Work out the finished part from the listing and answer in its coordinate system (mm). A direction names the side the tool comes from. Round coordinates to 2 decimals unless told otherwise and drop trailing zeros. Order: outer loops, then holes, each group sorted by start corner. A loop starts at its lowest first (then second) coordinate and runs counter-clockwise, first axis right, second up. Notation, with made-up numbers: M 69.25,-12 L 110.25,-12 A36 ccw 110.25,23 Z; hole C 57,-22.75 d11. An arc over 180 degrees is marked long. Return JSON: item names as keys, results as strings.
from build123d import *

# Parameters (mm, degrees)
CYLINDER011_R             = 1
CYLINDER011_DEPTH         = 1
CYLINDER003_R             = 2.25
CYLINDER003_DEPTH         = 10
ARRAY_X_COUNT             = 2
ARRAY_X_PITCH             = 49.5
ARRAY_Z_COUNT             = 2
ARRAY_Z_PITCH             = 10
EXTRUDE003_DEPTH          = 20.2
CUT004_ROLL_ANGLE         = -90
CUT004_PLACEMENT_ANGLE    = 90
FUSION002_PLACEMENT_ANGLE = 7


with BuildPart() as cylinder011:
    # Cylinder011 → Cylinder011 (new body)
    with BuildSketch(Plane(origin=(80, 0, -1), x_dir=(1, 0, 0), z_dir=(0, 0, 1))):
        Circle(CYLINDER011_R)
    extrude(amount=CYLINDER011_DEPTH)


with BuildPart() as array:
    # Cylinder003 → Cylinder003 (new body)
    with BuildSketch(Plane.XZ):
        Circle(CYLINDER003_R)
    extrude(amount=CYLINDER003_DEPTH)

    # Array X: Array ×2


with BuildPart() as array_1:
    add(array.part)
    with Locations(*[(i * ARRAY_X_PITCH, 0, 0) for i in range(1, ARRAY_X_COUNT)]):
        add(array.part)

    # Array Z: Array ×2


with BuildPart() as array_2:
    add(array_1.part)
    with Locations(*[(0, 0, i * ARRAY_Z_PITCH) for i in range(1, ARRAY_Z_COUNT)]):
        add(array_1.part)


with BuildPart() as array_3:
    # Array placement: moved
    add(array_2.part.moved(Location((-56.5, 22, 5))))


with BuildPart() as servo_pan:
    # Sketch002 → Extrude003 (new body)
    with BuildSketch(Plane.XY):
        Polygon((-59.135985, 19.221684), (-52.235985, 19.221684), (-52.235985, 27.421684), (-11.035985, 27.421684), (-11.035985, 19.221684), (-4.135985, 19.221684), (-4.135985, 16.721684), (-11.035985, 16.721684), (-11.035985, -10.278316), (-52.235985, -10.278316), (-52.235985, 16.721684), (-59.135985, 16.721684), align=None)
    extrude(amount=EXTRUDE003_DEPTH)

    # Cut004: cut Array
    add(array_3.part, mode=Mode.SUBTRACT)


with BuildPart() as servo_pan_1:
    # Cut004 roll: moved
    add(servo_pan.part.rotate(Axis((0, 0, 0), (1, 0, 0)), CUT004_ROLL_ANGLE))


with BuildPart() as servo_pan_2:
    # Cut004 placement: moved
    add(servo_pan_1.part.moved(Location((90, 21, 27))).rotate(Axis((90, 21, 27), (0, 0, 1)), CUT004_PLACEMENT_ANGLE))

    # Fusion002: union Cylinder011
    add(cylinder011.part)


with BuildPart() as servo_pan_3:
    # Fusion002 placement: moved
    add(servo_pan_2.part.moved(Location((0.6, 9.75, 0))).rotate(Axis((0.6, 9.75, 0), (0, 0, -1)), FUSION002_PLACEMENT_ANGLE))


solid = servo_pan_3.part
Item 1: Which of the six approach directions +Z, -Z, +X, -X, +Y, -Y give full straight-line access (tool end or side, diameter ignored) to faces 1 (the cylindrical face through (80.874, -0.492, -0.715)), 2 (the flat face through (82, 13, 10.278)), 3 (the flat face through (76, -34, 10.278)), 4 (the flat face through (82, 13, 7.778))?
Output:
{"face 1": "-Z", "face 2": "+Z, +X, +Y", "face 3": "+Z, -X, -Y", "face 4": "-Z, +X, +Y"}
Item 2: Find section A-A (x = 88.25). Determine the outline of the cut face in (y, z).
Output:
{"outline": "M -14.89,-0.42 L 9.03,-0.42 L 9.03,7.78 L 11.68,7.78 L 11.68,10.28 L 9.03,10.28 L 9.03,37.28 L -14.89,37.28 Z; M 14.89,7.78 L 15.98,7.78 L 15.98,10.28 L 14.89,10.28 Z"}
Item 3: Consider line 1 along Z through (x, y) = (74, -21); line 2 along Z through (x, y) = (80.5, 11); line 3 along Y through (x, z) = (75, 18.5). Determine where each line is inside the solid, lowest interval first. Write a range as [from, to].
Output:
{"line 1": "z = [-0.42, 37.28]", "line 2": "z = [7.78, 10.28]", "line 3": "y = [-30.86, 10.65]"}
Item 4: The mould has two halves that part along X. Classify faces 5 (the flat face through (68.63, -8.93, 18.16)), 6 (the flat face through (79, -11, -0.422)), 7 (the cylindrical face through (75.011, 15.937, 9.011)), 8 (the flat face through (81.259, 9.885, 23.589)): pulls with the +X half, pulls with the -X half, needs draft (parallel to the pull), parting line crosses it, or undercut.
Output:
{"face 5": "pulls with the -X half", "face 6": "needs draft", "face 7": "undercut", "face 8": "pulls with the +X half"}
Item 5: Find section D-D (x = 79.75). Determine the outline of the cut face in (y, z).
Output:
{"outline": "M -38.39,7.78 L -37.91,7.78 L -37.91,10.28 L -38.39,10.28 Z; M -33.78,7.78 L -31.44,7.78 L -31.44,-0.42 L -0.97,-0.42 L -0.97,-1 L 0.97,-1 L 0.97,-0.42 L 10.07,-0.42 L 10.07,7.78 L 17.02,7.78 L 17.02,10.28 L 10.07,10.28 L 10.07,37.28 L -31.44,37.28 L -31.44,10.28 L -33.78,10.28 Z"}
Item 6: Find section B-B (y = -35). Determine the outline of the cut face in (x, z).
Output:
{"outline": "M 65.43,7.78 L 68.5,7.78 L 68.5,10.28 L 65.43,10.28 Z; M 72.93,7.78 L 78.55,7.78 L 78.55,10.28 L 72.93,10.28 Z; M 82.73,7.78 L 85.78,7.78 L 85.78,10.28 L 82.73,10.28 Z"}
Item 7: Each of these flat-tipped pins is pushed along its axis until it touches: pin 1 (1.5 mm diameter, centred on y = -32, z = 9.5, fed in from +X); pin 2 (3 mm diameter, centred on x = 79, y = 6.5, fed in from -Z); pin 3 (1 mm diameter, centred on y = -21, z = 20, fed in from +X). Where does it stop, or does it pass through?
Output:
{"pin 1": "stops at x = 86.24", "pin 2": "stops at z = -0.42", "pin 3": "stops at x = 87.56"}
Item 8: Find section C-C (z = 13). Determine the outline of the cut face in (x, y).
Output:
{"outline": "M 66.07,-29.76 L 86.12,-32.22 L 91.14,8.67 L 71.09,11.13 Z"}
